```python
from build123d import *

# Parameters (mm, degrees)
F1_R             = 125
F4_DEPTH         = 5
F5_DEPTH         = 5
F5_COPIES_COUNT  = 6
F6_DEPTH         = 5
F6_COPIES_COUNT  = 6
F0_R             = 25
F7_DEPTH         = 25
F8_R             = 4
F9_DEPTH         = 5
F9_COPIES_COUNT  = 6
F10_R            = 3.5
F11_DEPTH        = 5
F11_COPIES_COUNT = 12


# Not quite as in the source:
# - a pattern or mirror of a feature is missing from the dataset's text; its kind, count and spacing are read off the source's solid


with BuildPart() as f4:
    # F1 (on Top) → F4 (new body)
    with BuildSketch(Plane.XY):
        Circle(F1_R)
    extrude(amount=-F4_DEPTH)

    # F2 (on Top) → F5 (cut, through all)
    with BuildSketch(Plane.XY):
        with BuildLine():
            ThreePointArc((15.75, 103.8120296497), (11.7403987974, 102.6600373885), (10, 98.8685996664))
            Line((10, 98.8685996664), (10, 47.6969600708))
            ThreePointArc((10, 47.6969600708), (10.9688711259, 44.7389201793), (13.5, 42.9272640638))
            ThreePointArc((13.5, 42.9272640638), (22.5, 38.9711431703), (30.4261011942, 33.154974983))
            ThreePointArc((30.4261011942, 33.154974983), (33.2606058502, 31.8687811355), (36.3067791046, 32.5087340733))
            Line((36.3067791046, 32.5087340733), (80.6227189477, 58.0945538711))
            ThreePointArc((80.6227189477, 58.0945538711), (83.0360009332, 61.4975023033), (82.0288548951, 65.5459149345))
            ThreePointArc((82.0288548951, 65.5459149345), (52.5, 90.9326673974), (15.75, 103.8120296497))
        make_face()
    f5 = extrude(amount=-F5_DEPTH, mode=Mode.SUBTRACT)

    # F5_copies: F5 ×6 about axis
    f5_copies_axis = Axis((0, 0, 0), (0, 0, 1))
    for i in range(1, F5_COPIES_COUNT):
        add(f5.rotate(f5_copies_axis, i * 360 / F5_COPIES_COUNT), mode=Mode.SUBTRACT)

    # F3 (on Top) → F6 (join, through all)
    with BuildSketch(Plane.XY):
        with BuildLine():
            Line((-10, 135), (-10, 120))
            Line((-10, 120), (10, 120))
            Line((10, 120), (10, 135))
            ThreePointArc((10, 135), (0, 145), (-10, 135))
        make_face()
    f6 = extrude(amount=-F6_DEPTH)

    # F6_copies: F6 ×6 about axis
    f6_copies_axis = Axis((0, 0, 0), (0, 0, 1))
    for i in range(1, F6_COPIES_COUNT):
        add(f6.rotate(f6_copies_axis, i * 360 / F6_COPIES_COUNT))

    # F0 (on Top) → F7 (cut)
    with BuildSketch(Plane.XY):
        Circle(F0_R)
    extrude(amount=-F7_DEPTH, mode=Mode.SUBTRACT)

    # F8 (on Top) → F9 (cut, through all)
    with BuildSketch(Plane.XY):
        with Locations((0, 135)):
            Circle(F8_R)
    f9 = extrude(amount=-F9_DEPTH, mode=Mode.SUBTRACT)

    # F9_copies: F9 ×6 about axis
    f9_copies_axis = Axis((0, 0, 0), (0, 0, 1))
    for i in range(1, F9_COPIES_COUNT):
        add(f9.rotate(f9_copies_axis, i * 360 / F9_COPIES_COUNT), mode=Mode.SUBTRACT)

    # F10 (on Top) → F11 (cut, through all)
    with BuildSketch(Plane.XY):
        with Locations((0, 115)):
            Circle(F10_R)
    f11 = extrude(amount=-F11_DEPTH, mode=Mode.SUBTRACT)

    # F11_copies: F11 ×12 about axis
    f11_copies_axis = Axis((0, 0, 0), (0, 0, 1))
    for i in range(1, F11_COPIES_COUNT):
        add(f11.rotate(f11_copies_axis, i * 360 / F11_COPIES_COUNT), mode=Mode.SUBTRACT)


solid = f4.part
```
Part model, mm, in its own coordinate system. Give positions to 0.01 mm unless a question says otherwise; leave off trailing zeros. Order: outer loops, then holes, each group sorted by start corner. A loop starts at its lowest first (then second) coordinate and runs counter-clockwise, first axis right, second up. Notation, with made-up numbers: (-17.75, 28) - (29.25, 28) arc R22 cw to (29.25, 50) - close; hole circle Ø8 at (59, 17.5). An arc over 180 degrees is marked (long way). Use one line per item in the form item = value.
Item 1: Slice it at C-C on y = -88. Give the cut face in (x, z) (3 decimals).
Solution:
outline = (-88.775, -5) - (-57.28, -5) - (-57.28, 0) - (-88.775, 0) - close; (-10, -5) - (10, -5) - (10, 0) - (-10, 0) - close; (57.28, -5) - (88.775, -5) - (88.775, 0) - (57.28, 0) - close
Item 2: Slice it at B-B on x = 0. Give the cut face in (y, z), and give its area (3 significant figures).
Solution:
outline = (-145, -5) - (-139, -5) - (-139, 0) - (-145, 0) - close; (-131, -5) - (-118.5, -5) - (-118.5, 0) - (-131, 0) - close; (-111.5, -5) - (-25, -5) - (-25, 0) - (-111.5, 0) - close; (25, -5) - (111.5, -5) - (111.5, 0) - (25, 0) - close; (118.5, -5) - (131, -5) - (131, 0) - (118.5, 0) - close; (139, -5) - (145, -5) - (145, 0) - (139, 0) - close
area = 1,050 mm2
Item 3: Pin check, flat tips, straight feed: pin 1 Ø1 at (x, z) = (74, -3.5) entering from -Y; pin 2 Ø6.5 at (x, y) = (99.59, -57.5) entering from +Z; pin 3 Ø2.5 at (y, z) = (65, -3) entering from -X (3 decimals); pin 4 Ø8 at (x, y) = (-57.5, 99.59) entering from +Z. Stop position of each tip, or through.
Solution:
pin_1 = -101.11
pin_2 = through
pin_3 = -126.835
pin_4 = 0
Item 4: Probe probe 1 along Y at (x, z) = (0, -3.45); probe 2 along X at (y, z) = (32.5, -1.45); probe 3 along X at (y, z) = (95.5, -0.55). List the from-to ranges inside material, lowest first. Write a range as from..to.
Solution:
probe_1 = -145..-139, -131..-118.5, -111.5..-25, 25..111.5, 118.5..131, 139..145
probe_2 = -120.7..-99.84, -76.29..-36.29, -31.32..31.32, 36.29..76.29, 99.84..120.7
probe_3 = -80.65..-43.64, -10..10, 43.64..80.65
Item 5: Two-plate mould, pull along Y, no slides. Class faces 1 (the face through (15, -22, -5)), 2 (the face through (125.68, 72.31, -2.46)), 3 (the face through (0, 145, -2)), 4 (the face through (-103.09, -57.35, -2.46)): released by +Y, released by -Y, zero draft, split by the parting line, or undercut.
Solution:
face_1 = zero draft
face_2 = undercut
face_3 = released by +Y
face_4 = undercut
Item 6: Slice it at A-A on y = 0. Give the cut face in (x, z).
Solution:
outline = (-125, -5) - (-118.5, -5) - (-118.5, 0) - (-125, 0) - close; (-111.5, -5) - (-105, -5) - (-105, 0) - (-111.5, 0) - close; (-45, -5) - (-25, -5) - (-25, 0) - (-45, 0) - close; (25, -5) - (45, -5) - (45, 0) - (25, 0) - close; (105, -5) - (111.5, -5) - (111.5, 0) - (105, 0) - close; (118.5, -5) - (125, -5) - (125, 0) - (118.5, 0) - close
